Here's the drawing with two shaded views (mm, measured from the low corner). I have some questions. A direction names the side the tool comes from. Round coordinates to 2 decimals unless told otherwise and drop trailing zeros. Loops run counter-clockwise (first coordinate to the right, second up) from the corner with the lowest first, then second, coordinate; pieces in that order, holes last. Notation, with made-up numbers: M 33.5,69 L 61.5,69 A29 cw 61.5,93 Z; hole C -13.75,37 d9. An arc over 180 degrees is marked long. One line per item, written item: value. Start each with the question number.
Q1. Please list where these lines run through material, in increasing order: line 1 along Y through (x, z) = (6, 1.3) (3 decimals); line 2 along Z through (x, y) = (1.25, 9.5); line 3 along Y through (x, z) = (7, 4).
Q2. I'm going to push flat-ended pins straight in: pin 1 Ø1 at (y, z) = (1.5, 2.5) entering from -X; pin 2 Ø2.5 at (y, z) = (5.5, 3) entering from -X. Where does each tip first touch, or does it pass through?
Q3. Imagine slicing it at C-C (z = 2.5). Please give me the cut outline in (x, y) (3 decimals).
Q4. Thinking about a two-plate mould opening in Y: for the marked faces 1, 2 and 3, which applies, released by +Y, released by -Y, zero draft, split by the parting line, or undercut?
Q5. Imagine slicing it at A-A (x = 6). Please give me the cut outline in (y, z) (3 decimals), then the cut area to 3 significant figures.
Q6. Which directions (+Z, -Z, +X, -X, +Y, -Y) give clear straight access to the entire face, cutting with the end or side of a thin tool? Please do the marked faces 4, 5, 6 and 7.
Q7. Imagine slicing it at B-B (y = 6). Please give me the cut outline in (x, z) (3 decimals), then the cut area to 3 significant figures.
Q8. Imagine slicing it at D-D (z = 1). Please give me the cut outline in (x, y) (3 decimals), then the cut area to 4 significant figures.
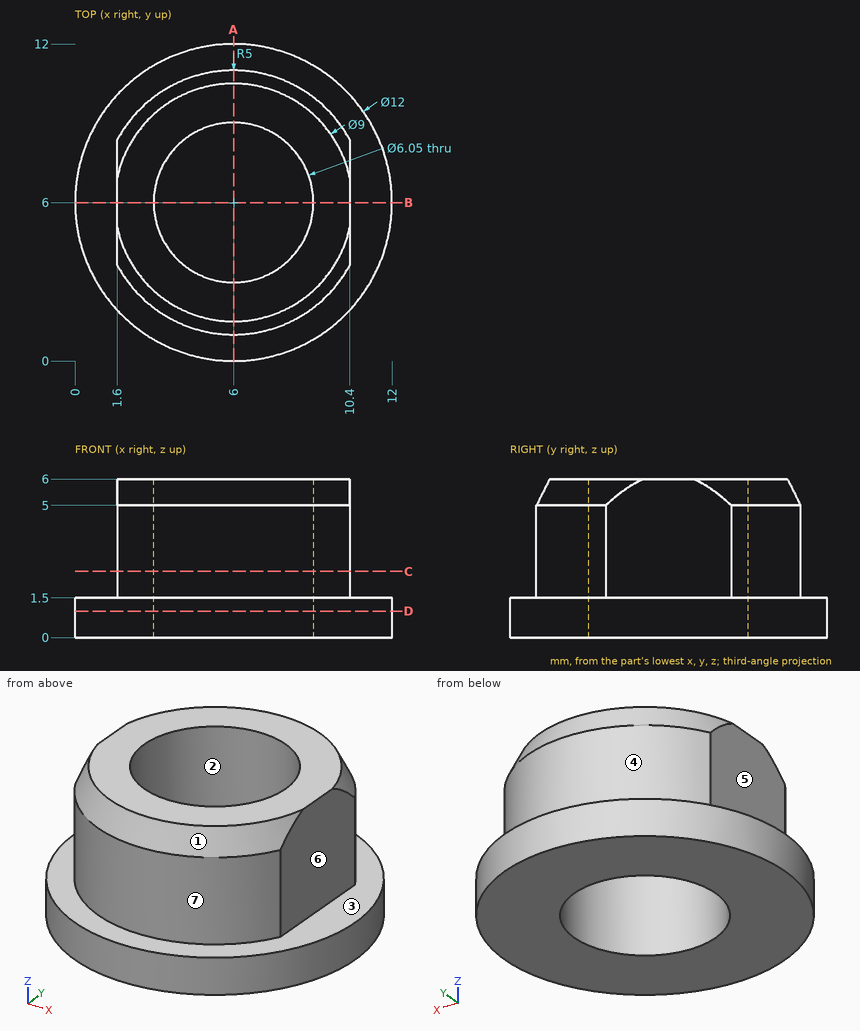
Report:
1. line 1: y = 0 to 2.975, 9.025 to 12
1. line 2: z = 0 to 1.5
1. line 3: y = 1.1 to 3.15, 8.85 to 10.9
2. pin 1: stops at x = 3
2. pin 2: stops at x = 1.6
3. outline: M 1.6,3.625 A5 ccw 10.4,3.625 L 10.4,8.375 A5 ccw 1.6,8.375 Z; hole C 6,6 d6.05
4. face 1: released by -Y
4. face 2: undercut
4. face 3: zero draft
5. outline: M 0,0 L 2.975,0 L 2.975,6 L 1.5,6 L 1,5 L 1,1.5 L 0,1.5 Z; M 9.025,0 L 12,0 L 12,1.5 L 11,1.5 L 11,5 L 10.5,6 L 9.025,6 Z
5. area: 26.2 mm²
6. face 4: +Z, +Y
6. face 5: +Z, -X, +Y, -Y
6. face 6: +Z, +X, +Y, -Y
6. face 7: +Z, -Y
7. outline: M 0,0 L 2.975,0 L 2.975,6 L 1.6,6 L 1.6,1.5 L 0,1.5 Z; M 9.025,0 L 12,0 L 12,1.5 L 10.4,1.5 L 10.4,6 L 9.025,6 Z
7. area: 21.3 mm²
8. outline: C 6,6 d12; hole C 6,6 d6.05
8. area: 84.35 mm²
